Geometry check sheet. Reference: the model listing, model coordinates, mm. Face numbers are marked on the shaded views. Round coordinates to 2 decimals unless told otherwise and drop trailing zeros. Write each loop counter-clockwise with the first axis right and the second up, starting at its lowest first coordinate (ties: lowest second). Pieces come first, ordered by that corner, then holes. Notation, with made-up numbers: (77.5, 9) - (104.5, 9) arc R6 ccw to (104.5, 20) - close; hole circle Ø3 at (26, 68). An arc over 180 degrees is marked (long way). One line per question, with ' | ' between items. Start each with the question number.
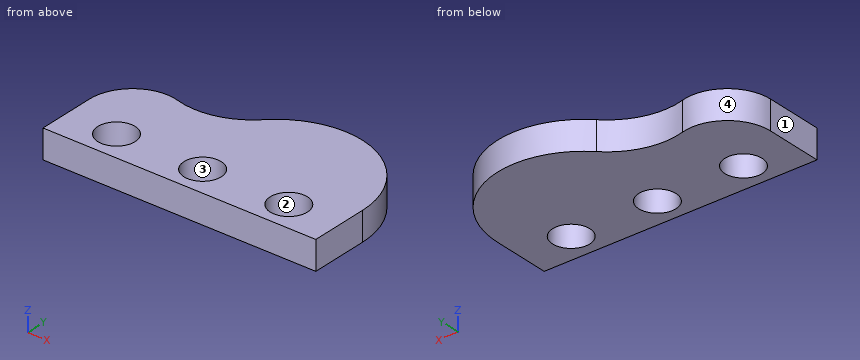
from build123d import *

# Parameters (mm, degrees)
SKETCH1_R           = 6.5
BOSS_EXTRUDE1_DEPTH = 5


with BuildPart() as part:
    # Sketch1 → Boss-Extrude1 (new body, symmetric)
    with BuildSketch(Plane.XY):
        with BuildLine():
            Line((0, 20), (0, 0))
            Line((0, 0), (95, 0))
            Line((95, 0), (95, 20))
            ThreePointArc((95, 20), (76.35181203, 47.769342153), (43.590909091, 41.015490155))
            ThreePointArc((43.590909091, 41.015490155), (32.208180594, 34.376961736), (19.03125, 34.448149481))
            ThreePointArc((19.03125, 34.448149481), (5.929960033, 31.947149242), (0, 20))
        make_face()
        with Locations((17.5, 10)):
            Circle(SKETCH1_R, mode=Mode.SUBTRACT)
        with Locations((47.5, 10)):
            Circle(SKETCH1_R, mode=Mode.SUBTRACT)
        with Locations((77.5, 10)):
            Circle(SKETCH1_R, mode=Mode.SUBTRACT)
    extrude(amount=BOSS_EXTRUDE1_DEPTH, both=True)


solid = part.part
Q1. Thickness scan on line 1 (X direction, y = 13.5, z = 3.5); line 2 (X direction, y = 15, z = 0); line 3 (Y direction, x = 47.5, z = 0.25). Record the ranges inside material, lowest first.
Q2. Section check B-B, the plane x = 47.5. Record the cut outline in (y, z).
Q3. Section check C-C, the plane z = -0.75. Record the cut outline in (x, y), then the cut area to 3 significant figures.
Q4. Go/stop test with flat-tipped pins: P1, Ø2, axis at y = 22, z = 1, coming from the +X side; P2, Ø21, axis at x = 77.5, y = 10, coming from the -Z side; P3, Ø10.5, axis at x = 17.5, y = 10, coming from the -Z side; P4, Ø5, axis at x = 41.5, z = 2.5, coming from the +Y side. Record where each tip stops, or that it passes through.
Q5. Section check D-D, the plane x = 17.5. Record the cut outline in (y, z).
Q6. Draft check along Y on the marked faces 1, 2, 3 and 4. Enter one of: pulls with the +Y half, pulls with the -Y half, needs draft (parallel to the pull), parting line crosses it, or undercut.
Q7. Section check A-A, the plane y = 10. Record the cut outline in (x, z).
Result sheet:
1) line 1: 0 to 12.02, 22.98 to 42.02, 52.98 to 72.02, 82.98 to 95 | line 2: 0 to 13.35, 21.65 to 43.35, 51.65 to 73.35, 81.65 to 95 | line 3: 0 to 3.5, 16.5 to 44.37
2) outline: (0, -5) - (3.5, -5) - (3.5, 5) - (0, 5) - close; (16.5, -5) - (44.37, -5) - (44.37, 5) - (16.5, 5) - close
3) outline: (0, 0) - (95, 0) - (95, 20) arc R30 ccw to (43.59, 41.02) arc R25 cw to (19.03, 34.45) arc R15 ccw to (0, 20) - close; hole circle Ø13 at (17.5, 10); hole circle Ø13 at (47.5, 10); hole circle Ø13 at (77.5, 10) | area: 3,400 mm²
4) P1: x = 94.98 | P2: z = -5 | P3: through | P4: y = 41.42
5) outline: (0, -5) - (3.5, -5) - (3.5, 5) - (0, 5) - close; (16.5, -5) - (34.79, -5) - (34.79, 5) - (16.5, 5) - close
6) face 1: needs draft | face 2: undercut | face 3: undercut | face 4: pulls with the +Y half
7) outline: (0, -5) - (11, -5) - (11, 5) - (0, 5) - close; (24, -5) - (41, -5) - (41, 5) - (24, 5) - close; (54, -5) - (71, -5) - (71, 5) - (54, 5) - close; (84, -5) - (95, -5) - (95, 5) - (84, 5) - close
